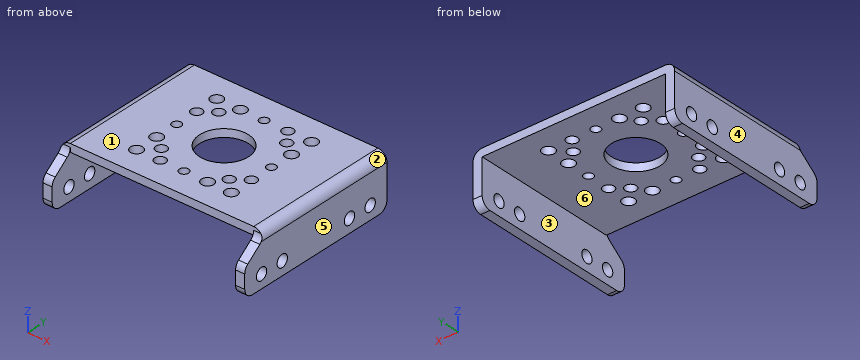
```python
from build123d import *

# Parameters (mm, degrees)
SKETCH1_W           = 33
SKETCH1_H           = 24
SKETCH1_R           = 4
SKETCH1_R_2         = 1
SKETCH1_R_3         = 0.75
SKETCH1_R_4         = 0.9
BOSS_EXTRUDE1_DEPTH = 1.3
SKETCH2_R           = 1
BOSS_EXTRUDE2_DEPTH = 1.5
FILLET1_R           = 1.5


with BuildPart() as part:
    # Sketch1 → Boss-Extrude1 (new body)
    with BuildSketch(Plane.XY):
        Rectangle(SKETCH1_W, SKETCH1_H)
        Circle(SKETCH1_R, mode=Mode.SUBTRACT)
        with Locations((-7.75, 7.75)):
            Circle(SKETCH1_R_2, mode=Mode.SUBTRACT)
        with Locations((7.75, 7.75)):
            Circle(SKETCH1_R_2, mode=Mode.SUBTRACT)
        with Locations((7.75, -7.75)):
            Circle(SKETCH1_R_2, mode=Mode.SUBTRACT)
        with Locations((-7.75, -7.75)):
            Circle(SKETCH1_R_2, mode=Mode.SUBTRACT)
        with Locations((0, 7.75)):
            Circle(SKETCH1_R_3, mode=Mode.SUBTRACT)
        with Locations((-3.875, 7.75)):
            Circle(SKETCH1_R_2, mode=Mode.SUBTRACT)
        with Locations((3.88, 7.75)):
            Circle(SKETCH1_R_4, mode=Mode.SUBTRACT)
        with Locations((-5.557968978, 5.557968978)):
            Circle(SKETCH1_R_4, mode=Mode.SUBTRACT)
        with Locations((7.75, 3.875)):
            Circle(SKETCH1_R_2, mode=Mode.SUBTRACT)
        with Locations((7.75, 0)):
            Circle(SKETCH1_R_3, mode=Mode.SUBTRACT)
        with Locations((7.75, -3.88)):
            Circle(SKETCH1_R_4, mode=Mode.SUBTRACT)
        with Locations((5.557968978, 5.557968978)):
            Circle(SKETCH1_R_4, mode=Mode.SUBTRACT)
        with Locations((3.875, -7.75)):
            Circle(SKETCH1_R_2, mode=Mode.SUBTRACT)
        with Locations((0, -7.75)):
            Circle(SKETCH1_R_3, mode=Mode.SUBTRACT)
        with Locations((-3.88, -7.75)):
            Circle(SKETCH1_R_4, mode=Mode.SUBTRACT)
        with Locations((5.557968978, -5.557968978)):
            Circle(SKETCH1_R_4, mode=Mode.SUBTRACT)
        with Locations((-7.75, -3.875)):
            Circle(SKETCH1_R_2, mode=Mode.SUBTRACT)
        with Locations((-7.75, 0)):
            Circle(SKETCH1_R_3, mode=Mode.SUBTRACT)
        with Locations((-7.75, 3.88)):
            Circle(SKETCH1_R_4, mode=Mode.SUBTRACT)
        with Locations((-5.557968978, -5.557968978)):
            Circle(SKETCH1_R_4, mode=Mode.SUBTRACT)
    extrude(amount=BOSS_EXTRUDE1_DEPTH)

    # Sketch2 → Boss-Extrude2 (add)
    with BuildSketch(Plane(origin=(16.5, 0, 0), x_dir=(0, 0, -1), z_dir=(1, 0, 0))):
        with BuildLine():
            Line((5.7, 12), (0, 12))
            Line((0, 12), (0, -12))
            Line((0, -12), (-0.73731738, -12))
            ThreePointArc((-0.73731738, -12), (-0.075617967, -12.153837348), (0.450356003, -12.583794819))
            Line((0.450356003, -12.583794819), (2.249643997, -14.916205181))
            ThreePointArc((2.249643997, -14.916205181), (2.775617967, -15.346162652), (3.43731738, -15.5))
            Line((3.43731738, -15.5), (5.7, -15.5))
            ThreePointArc((5.7, -15.5), (6.760660172, -15.060660172), (7.2, -14))
            Line((7.2, -14), (7.2, 10.5))
            ThreePointArc((7.2, 10.5), (6.760660172, 11.560660172), (5.7, 12))
        make_face()
        with Locations((4.98, -12.25)):
            Circle(SKETCH2_R, mode=Mode.SUBTRACT)
        with Locations((4.98, -8.25)):
            Circle(SKETCH2_R, mode=Mode.SUBTRACT)
        with Locations((4.98, 4.75)):
            Circle(SKETCH2_R, mode=Mode.SUBTRACT)
        with Locations((4.98, 8.75)):
            Circle(SKETCH2_R, mode=Mode.SUBTRACT)
    boss_extrude2 = extrude(amount=-BOSS_EXTRUDE2_DEPTH)

    # Mirror1: Boss-Extrude2 across plane
    add(boss_extrude2.mirror(Plane(origin=(0, 0, 0), x_dir=(0, 0, 1), z_dir=(1, 0, 0))))

    # Fillet1
    fillet1_edges = [part.edges().sort_by_distance(p)[0] for p in [
        (-16.5, 0, 1.3),
        (16.5, 0, 1.3),
    ]]
    fillet(fillet1_edges, radius=FILLET1_R)


solid = part.part
```
Build history of the part. All positions in model axes, mm. Face numbers are marked on the shaded views. A direction names the side the tool comes from. Round coordinates to 2 decimals unless told otherwise and drop trailing zeros. Loops run counter-clockwise (first coordinate to the right, second up) from the corner with the lowest first, then second, coordinate; pieces in that order, holes last. Notation, with made-up numbers: M 70.5,-5.75 L 102.5,-5.75 A11 cw 102.5,10.25 Z; hole C 13,69.25 d10. An arc over 180 degrees is marked long. Answer as CSV lines item,"result".
1. Cut at B-B on x = -6. Write the cut outline in (y, z).
Resolved:
outline,"M -12,0 L -6.34,0 L -6.34,1.3 L -12,1.3 Z; M -4.77,0 L 4.77,0 L 4.77,1.3 L -4.77,1.3 Z; M 6.34,0 L 12,0 L 12,1.3 L 6.34,1.3 Z"
2. Cut at D-D on x = 9.5. Write the cut outline in (y, z).
Resolved:
outline,"M -12,0 L 12,0 L 12,1.3 L -12,1.3 Z"
3. Cut at C-C on z = -6.5. Write the cut outline in (x, y), then the cut area to 3 significant figures.
Resolved:
outline,"M -16.5,-15.27 L -15,-15.27 L -15,11.77 L -16.5,11.77 Z; M 15,-15.27 L 16.5,-15.27 L 16.5,11.77 L 15,11.77 Z"
area,"81.1 mm²"
4. 3-axis set-ups, long thin cutter, end or side, ignore diameter. For the marked faces 5 and 6: which of +Z, -Z, +X, -X, +Y, -Y reach the whole face in a straight line?
Resolved:
face 5,"+Z, -Z, +X, +Y, -Y"
face 6,"-Z, +Y, -Y"
5. Two-plate mould, pull along X, no slides. Class the marked faces 1, 2, 3 and 4: released by +X, released by -X, zero draft, split by the parting line, or undercut.
Resolved:
face 1,"zero draft"
face 2,"released by +X"
face 3,"undercut"
face 4,"released by -X"
6. Flat gauge pin, fed straight in: P1, Ø2.5, axis at x = 0, y = -7.75, coming from the -Z side. Where does the tip first touch, or does it go through?
Resolved:
P1,"stops at z = 0"
7. Cut at A-A on y = -1.75. Write the cut outline in (x, z).
Resolved:
outline,"M -16.5,-7.2 L -15,-7.2 L -15,0 L -3.6,0 L -3.6,1.3 L -15,1.3 A1.5 ccw -16.5,-0.2 Z; M 3.6,0 L 15,0 L 15,-7.2 L 16.5,-7.2 L 16.5,-0.2 A1.5 ccw 15,1.3 L 3.6,1.3 Z"
8. Wall check: probe 1 along Y at (x, z) = (-7.75, 0.45) (3 decimals); probe 2 along X at (y, z) = (-1.5, -1.5); probe 3 along Z at (x, y) = (10.5, -2). Give the ranges that are in metal, low to high. Write a range as [from, to].
Resolved:
probe 1,"y = [-12, -8.75], [-6.75, -4.875], [-2.875, -0.75], [0.75, 2.98], [4.78, 6.75], [8.75, 12]"
probe 2,"x = [-16.5, -15], [15, 16.5]"
probe 3,"z = [0, 1.3]"
